from build123d import *

# Parameters (mm, degrees)
SKETCH1_W           = 202.7
SKETCH1_H           = 137.7
SKETCH1_W_2         = 190
SKETCH1_H_2         = 125
BOSS_EXTRUDE1_DEPTH = 65
SKETCH2_W           = 202.7
SKETCH2_H           = 137.7
BOSS_EXTRUDE2_DEPTH = 6.35
CUT_EXTRUDE1_REACH  = 225.724
SKETCH3_R           = 8
SKETCH4_W           = 215.4
SKETCH4_H           = 150.4
SKETCH4_W_2         = 202.7
SKETCH4_H_2         = 137.7
BOSS_EXTRUDE3_DEPTH = 15
SKETCH5_W           = 215.4
SKETCH5_H           = 150.4
BOSS_EXTRUDE4_DEPTH = 25.4


with BuildPart() as part:
    # Sketch1 → Boss-Extrude1 (new body)
    with BuildSketch(Plane(origin=(0, 0, 0), x_dir=(1, 0, 0), z_dir=(0, 1, 0))):
        Rectangle(SKETCH1_W, SKETCH1_H)
        Rectangle(SKETCH1_W_2, SKETCH1_H_2, mode=Mode.SUBTRACT)
    extrude(amount=BOSS_EXTRUDE1_DEPTH)

    # Sketch2 → Boss-Extrude2 (add)
    with BuildSketch(Plane.XZ):
        Rectangle(SKETCH2_W, SKETCH2_H)
    extrude(amount=BOSS_EXTRUDE2_DEPTH)

    # Sketch3 → Cut-Extrude1 (cut, up to next)
    with BuildSketch(Plane.ZY.offset(-101.35), mode=Mode.PRIVATE) as cut_extrude1_sk1:
        with Locations((14.875, 33.25)):
            Circle(SKETCH3_R)
    cut_extrude1_tool1 = extrude(cut_extrude1_sk1.sketch, amount=CUT_EXTRUDE1_REACH, mode=Mode.PRIVATE) & part.part
    # Sketch3 → Cut-Extrude1 (cut, up to next)
    with BuildSketch(Plane.ZY.offset(-101.35), mode=Mode.PRIVATE) as cut_extrude1_sk2:
        with Locations((43.45, 33.25)):
            Circle(SKETCH3_R)
    cut_extrude1_tool2 = extrude(cut_extrude1_sk2.sketch, amount=CUT_EXTRUDE1_REACH, mode=Mode.PRIVATE) & part.part
    cut_extrude1_1 = cut_extrude1_tool1.solids().sort_by_distance((101.35, 33.25, 14.875))[0]
    add(cut_extrude1_1, mode=Mode.SUBTRACT)
    cut_extrude1_2 = cut_extrude1_tool2.solids().sort_by_distance((101.35, 33.25, 43.45))[0]
    add(cut_extrude1_2, mode=Mode.SUBTRACT)
    cut_extrude1 = cut_extrude1_1 + cut_extrude1_2  # Cut-Extrude1 as one shape, for the pattern or mirror that repeats it

    # Mirror1: Cut-Extrude1 across plane
    add(cut_extrude1.mirror(Plane.XY), mode=Mode.SUBTRACT)

    # Sketch4 → Boss-Extrude3 (add)
    with BuildSketch(Plane(origin=(0, 65, 0), x_dir=(1, 0, 0), z_dir=(0, 1, 0))):
        Rectangle(SKETCH4_W, SKETCH4_H)
        Rectangle(SKETCH4_W_2, SKETCH4_H_2, mode=Mode.SUBTRACT)
    extrude(amount=-BOSS_EXTRUDE3_DEPTH)

    # Sketch5 → Boss-Extrude4 (add)
    with BuildSketch(Plane(origin=(0, 65, 0), x_dir=(1, 0, 0), z_dir=(0, 1, 0))):
        Rectangle(SKETCH5_W, SKETCH5_H)
    extrude(amount=BOSS_EXTRUDE4_DEPTH)


solid = part.part
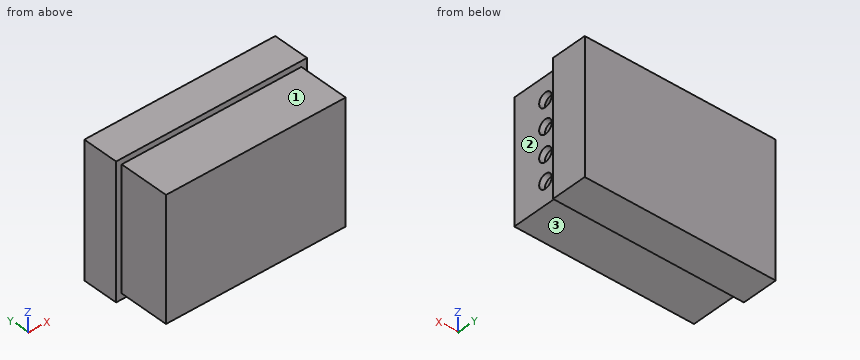
Check sheet for the modelled part. Datum: model origin and axes. Units: mm. Face numbers are marked on the shaded views. A direction names the side the tool comes from. Give positions to 0.01 mm unless a question says otherwise; leave off trailing zeros. Write each loop counter-clockwise with the first axis right and the second up, starting at its lowest first coordinate (ties: lowest second). Pieces come first, ordered by that corner, then holes. Notation, with made-up numbers: (75.25, 4) -> (119.25, 4) arc R12 cw to (119.25, 24) -> close; hole circle Ø8 at (20.5, -35.75). An arc over 180 degrees is marked (long way). Write item = value, one per line.
Item 1: Gauge pin test, flat ends, axial feed: pin 1 (17 mm diameter, centred on y = 11.5, z = 27, fed in from -X); pin 2 (10 mm diameter, centred on y = 15, z = 4.5, fed in from +X); pin 3 (17 mm diameter, centred on x = 30, y = 11, fed in from +Z). Record the tip position at first contact, or that the pin passes through.
Output:
pin_1 = -101.35
pin_2 = 101.35
pin_3 = 68.85
Item 2: Sectioned sample at A-A on y = 33.25. Record the boundary of the cut face in (x, z) (3 decimals), and give its area (3 significant figures).
Output:
outline = (-101.35, -68.85) -> (101.35, -68.85) -> (101.35, -51.45) -> (95, -51.45) -> (95, -62.5) -> (-95, -62.5) -> (-95, 62.5) -> (95, 62.5) -> (95, 51.45) -> (101.35, 51.45) -> (101.35, 68.85) -> (-101.35, 68.85) -> close; (95, -35.45) -> (101.35, -35.45) -> (101.35, -22.875) -> (95, -22.875) -> close; (95, -6.875) -> (101.35, -6.875) -> (101.35, 6.875) -> (95, 6.875) -> close; (95, 22.875) -> (101.35, 22.875) -> (101.35, 35.45) -> (95, 35.45) -> close
area = 3,760 mm^2
Item 3: Tool access check on the marked faces 1, 2 and 3. Record the directions out of +Z, -Z, +X, -X, +Y, -Y that give a thin tool (end or side, any length) a straight path to the whole face; none if there is none.
Output:
face_1 = +Z, +X, -X, -Y
face_2 = +Z, -Z, +X, -Y
face_3 = -Z, +X, -X, -Y
Item 4: Sectioned sample at C-C on y = 57. Record the boundary of the cut face in (x, z), and give its area (3 significant figures).
Output:
outline = (-107.7, -75.2) -> (107.7, -75.2) -> (107.7, 75.2) -> (-107.7, 75.2) -> close; hole (-95, -62.5) -> (95, -62.5) -> (95, 62.5) -> (-95, 62.5) -> close
area = 8,650 mm^2
Item 5: Sectioned sample at D-D on z = 58. Record the boundary of the cut face in (x, y), and give its area (3 significant figures).
Output:
outline = (-107.7, 50) -> (-101.35, 50) -> (-101.35, -6.35) -> (101.35, -6.35) -> (101.35, 50) -> (107.7, 50) -> (107.7, 90.4) -> (-107.7, 90.4) -> close; hole (-95, 0) -> (95, 0) -> (95, 65) -> (-95, 65) -> close
area = 7,770 mm^2
Item 6: Scan lines: probe 1 along Z at (x, y) = (97.25, 33.25) (3 decimals); probe 2 along Y at (x, z) = (70.5, 58); probe 3 along X at (y, z) = (64, -35.5). Record each from-to range of solid material in increasing order. Write a range as from..to.
Output:
probe_1 = -68.85..-51.45, -35.45..-22.875, -6.875..6.875, 22.875..35.45, 51.45..68.85
probe_2 = -6.35..0, 65..90.4
probe_3 = -107.7..-95, 95..107.7
Item 7: Sectioned sample at B-B on x = 25. Record the boundary of the cut face in (y, z), and give its area (3 significant figures).
Output:
outline = (-6.35, -68.85) -> (50, -68.85) -> (50, -75.2) -> (90.4, -75.2) -> (90.4, 75.2) -> (50, 75.2) -> (50, 68.85) -> (-6.35, 68.85) -> close; hole (0, -62.5) -> (65, -62.5) -> (65, 62.5) -> (0, 62.5) -> close
area = 5,710 mm^2
